```python
from build123d import *

# Parameters (mm, degrees)
SKETCH_1_R      = 32.5
SKETCH_1_R_2    = 22.779013497
EXTRUDE_1_DEPTH = 27
FILLET_1_R      = 2
FILLET_2_R      = 0.5
SKETCH_1_3_R    = 22.779013497
EXTRUDE_2_DEPTH = 15


with BuildPart() as part:
    # Sketch 1 → Extrude 1 (new body)
    with BuildSketch(Plane(origin=(0, 0, 0), x_dir=(1, 0, 0), z_dir=(0, 1, 0))):
        with Locations(Location((0, 0, 0), (0, 0, 270))):
            Circle(SKETCH_1_R)
        with Locations(Location((0, 0, 0), (0, 0, 270))):
            Circle(SKETCH_1_R_2, mode=Mode.SUBTRACT)
    extrude(amount=EXTRUDE_1_DEPTH)

    # Fillet 1
    fillet_1_edges = [part.edges().sort_by_distance(p)[0] for p in [
        (0, 0, -32.5),
        (0, 27, -32.5),
    ]]
    fillet(fillet_1_edges, radius=FILLET_1_R)

    # Fillet 2
    fillet_2_edges = [part.edges().sort_by_distance(p)[0] for p in [
        (0, 0, -22.779013497),
        (0, 27, -22.779013497),
    ]]
    fillet(fillet_2_edges, radius=FILLET_2_R)

    # Sketch 1_3 → Extrude 2 (add)
    with BuildSketch(Plane(origin=(0, 0, 0), x_dir=(1, 0, 0), z_dir=(0, 1, 0))):
        with Locations(Location((0, 0, 0), (0, 0, 270))):
            Circle(SKETCH_1_3_R)
    extrude(amount=EXTRUDE_2_DEPTH)


solid = part.part
```
Input: part model. Units: mm. Frame: model coordinates. A direction names the side the tool comes from. Round coordinates to 2 decimals unless told otherwise and drop trailing zeros. Loops run counter-clockwise (first coordinate to the right, second up) from the corner with the lowest first, then second, coordinate; pieces in that order, holes last. Notation, with made-up numbers: M 78,72.5 L 111,72.5 A34 cw 111,111.5 Z; hole C 52.25,64 d4. An arc over 180 degrees is marked long. Answer in a Markdown table with one row per item. Add a question column.
1. Section D-D (y = 10.75). Output: boundary loops of the cut face in (x, z), and give its area (3 significant figures).
2. Set-up query: faces 4 (the face through (-22.5, 0, -6.9)), 5 (the face through (19.207, 20.67, 12.246)). Return all of +Z, -Z, +X, -X, +Y, -Y with unobstructed straight access to the full face (end or side cutting, diameter ignored); none if empty.
3. Contact query for flat-ended pins moving along their axis: pin 1 (1 mm diameter, centred on x = -18.5, y = 20, fed in from -Z); pin 2 (5 mm diameter, centred on x = -24.5, y = 19, fed in from -Z); pin 3 (2 mm diameter, centred on x = 22, z = -15.5, fed in from -Y); pin 4 (6 mm diameter, centred on x = -18.5, y = 21, fed in from -Z). Output: stop coordinate, or through.
4. Mould query, pull axis X, two halves, no side actions, for faces 1 (the face through (0, 15, 0)), 2 (the face through (9.76, 13.34, 31)), 3 (the face through (0, 0, 0)). Classes: released by +X, released by -X, zero draft, split by the parting line, or undercut.
5. Section C-C (y = 17.75). Output: boundary loops of the cut face in (x, z), and give its area (3 significant figures).
6. Section B-B (x = 0). Output: boundary loops of the cut face in (y, z).
7. Ray query, probe 1 along X at (y, z) = (18, 0); probe 2 along Y at (x, z) = (-11, 11); probe 3 along Z at (x, y) = (0.5, 8). Return the intervals inside material, ascending.
8. Section A-A (z = 0). Output: boundary loops of the cut face in (x, y).
Values follow:
| question | item | result |
|---|---|---|
| 1 | outline | C 0,0 d65 |
| 1 | area | 3,320 mm^2 |
| 2 | face 4 | +Z, -Z, +X, -X, -Y |
| 2 | face 5 | +Y |
| 3 | pin 1 | z = -27.06 |
| 3 | pin 2 | z = -23.92 |
| 3 | pin 3 | y = 0 |
| 3 | pin 4 | z = -28.57 |
| 4 | face 1 | undercut |
| 4 | face 2 | split by the parting line |
| 4 | face 3 | zero draft |
| 5 | outline | C 0,0 d65; hole C 0,0 d45.56 |
| 5 | area | 1,690 mm^2 |
| 6 | outline | M 0,-30.5 A2 ccw 2,-32.5 L 25,-32.5 A2 ccw 27,-30.5 L 27,-23.28 A0.5 ccw 26.5,-22.78 L 15,-22.78 L 15,22.78 L 26.5,22.78 A0.5 ccw 27,23.28 L 27,30.5 A2 ccw 25,32.5 L 2,32.5 A2 ccw 0,30.5 L 0,23.28 A0.5 ccw 0.5,22.78 L 0,22.78 L 0,-22.78 L 0.5,-22.78 A0.5 ccw 0,-23.28 Z |
| 7 | probe 1 | -32.5 to -22.78, 22.78 to 32.5 |
| 7 | probe 2 | 0 to 15 |
| 7 | probe 3 | -32.5 to 32.5 |
| 8 | outline | M -32.5,2 A2 ccw -30.5,0 L -23.28,0 A0.5 ccw -22.78,0.5 L -22.78,0 L 22.78,0 L 22.78,0.5 A0.5 ccw 23.28,0 L 30.5,0 A2 ccw 32.5,2 L 32.5,25 A2 ccw 30.5,27 L 23.28,27 A0.5 ccw 22.78,26.5 L 22.78,15 L -22.78,15 L -22.78,26.5 A0.5 ccw -23.28,27 L -30.5,27 A2 ccw -32.5,25 Z |
